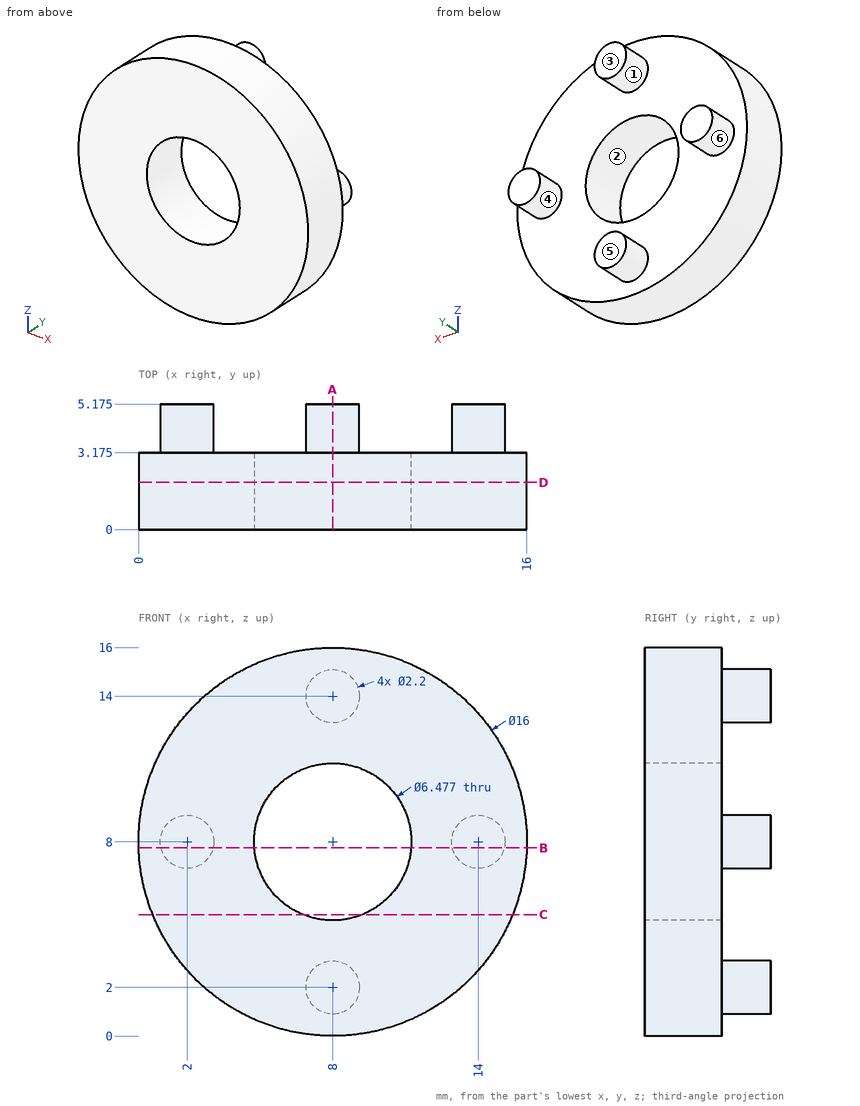
Design review of the part shown in the three views and the two pictorial views. Dimensions are in mm from the part's minimum x, y and z. A direction names the side the tool comes from. Coordinates: 2 decimals unless noted, no trailing zeros. Write each loop counter-clockwise with the first axis right and the second up, starting at its lowest first coordinate (ties: lowest second). Pieces come first, ordered by that corner, then holes.
(1) The part is to be moulded in two halves that separate along X. For the marked faces 1, 2, 3 and 4, say which applies: +X half, -X half, draft (parallel to the pull), parting line (faces both ways), or undercut.
(2) Wall thickness on probe 1 along Z at (x, y) = (8, 2.55); probe 2 along Z at (x, y) = (8, 3.85): over which ranges is each line inside the solid? List them lowest first.
(3) Add section B-B on z = 7.75. Give the boundary of the cut face in (x, y) (3 decimals), then the cut area to 3 significant figures.
(4) Add section A-A on x = 8. Give the boundary of the cut face in (y, z) (1 decimal).
(5) For pin 1 Ø4 at (x, z) = (13.5, 3) entering from +Y (3 decimals); pin 2 Ø1 at (x, y) = (10, 3) entering from -Z, all flat-tipped, find the tip position at first contact; note any pin that passes through.
(6) Add section D-D on y = 1.95. Give the boundary of the cut face in (x, z), then the cut area to 3 significant figures.
(7) Tool access review of the marked faces 5 and 6: name each direction out of +Z, -Z, +X, -X, +Y, -Y from which nothing blocks a thin tool from reaching the whole face with its end or side.
(8) Add section C-C on z = 5. Give the boundary of the cut face in (x, y) (3 decimals), then the cut area to 3 significant figures.
Answer sheet:
1. face 1: parting line
1. face 2: undercut
1. face 3: draft
1. face 4: undercut
2. probe 1: z = 0 to 4.76, 11.24 to 16
2. probe 2: z = 0.9 to 3.1, 12.9 to 15.1
3. outline: (0.004, 0) - (4.771, 0) - (4.771, 3.175) - (3.071, 3.175) - (3.071, 5.175) - (0.929, 5.175) - (0.929, 3.175) - (0.004, 3.175) - close; (11.229, 0) - (15.996, 0) - (15.996, 3.175) - (15.071, 3.175) - (15.071, 5.175) - (12.929, 5.175) - (12.929, 3.175) - (11.229, 3.175) - close
3. area: 38.8 mm2
4. outline: (0, 0) - (3.2, 0) - (3.2, 0.9) - (5.2, 0.9) - (5.2, 3.1) - (3.2, 3.1) - (3.2, 4.8) - (0, 4.8) - close; (0, 11.2) - (3.2, 11.2) - (3.2, 12.9) - (5.2, 12.9) - (5.2, 15.1) - (3.2, 15.1) - (3.2, 16) - (0, 16) - close
5. pin 1: stops at y = 3.175
5. pin 2: stops at z = 0.14
6. outline: circle Ø16 at (8, 8); hole circle Ø6.48 at (8, 8)
6. area: 168 mm2
7. face 5: +Z, -Z, +X, -X, +Y
7. face 6: +Y
8. outline: (0.584, 0) - (6.78, 0) - (6.78, 3.175) - (0.584, 3.175) - close; (9.22, 0) - (15.416, 0) - (15.416, 3.175) - (9.22, 3.175) - close
8. area: 39.3 mm2
